Input: part model. Units: mm. Frame: model coordinates. Face numbers are marked on the shaded views. A direction names the side the tool comes from. Round coordinates to 2 decimals unless told otherwise and drop trailing zeros. Write each loop counter-clockwise with the first axis right and the second up, starting at its lowest first coordinate (ties: lowest second). Pieces come first, ordered by that corner, then holes. Notation, with made-up numbers: (64, 57) - (98, 57) arc R25 cw to (98, 88) - close; hole circle Ø9 at (30.25, 23.5). An arc over 180 degrees is marked (long way). Use one line per item in the form item = value.
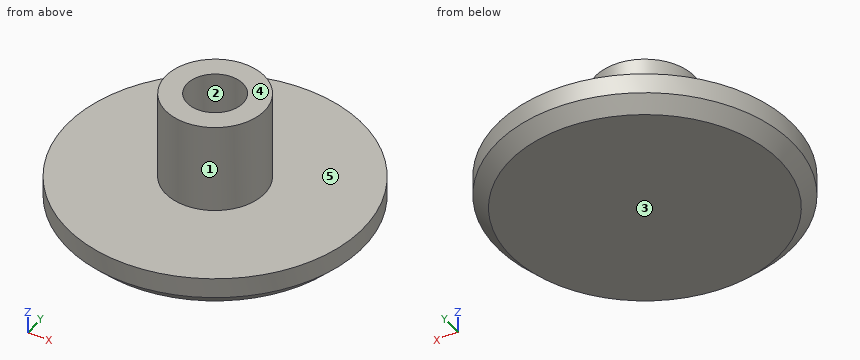
```python
from build123d import *

# Parameters (mm, degrees)
F0_R     = 11
F1_DEPTH = 2.5
F2_SIZE2 = 1
F2_SIZE  = 1
F3_R     = 3.675
F4_DEPTH = 6.6
F5_R     = 2.075
F6_DEPTH = 6


with BuildPart() as f1:
    # F0 (on Top) → F1 (new body)
    with BuildSketch(Plane.XY):
        Circle(F0_R)
    extrude(amount=F1_DEPTH)

    # F2
    f2_edges = [f1.edges().sort_by_distance(p)[0] for p in [
        (-11, 0, 0),
    ]]
    chamfer(f2_edges, length=F2_SIZE, length2=F2_SIZE2)

    # F3 (on face) → F4 (join)
    with BuildSketch(Plane.XY.offset(2.5)):
        Circle(F3_R)
    extrude(amount=F4_DEPTH)

    # F5 (on face) → F6 (cut)
    with BuildSketch(Plane.XY.offset(9.1)):
        Circle(F5_R)
    extrude(amount=-F6_DEPTH, mode=Mode.SUBTRACT)


solid = f1.part
```
(1) Draft query along Y for the marked faces 1, 2 and 3. Return one class per face: released by +Y, released by -Y, zero draft, split by the parting line, or undercut.
Derived:
face_1 = split by the parting line
face_2 = undercut
face_3 = zero draft
(2) Cut plane A-A on y = 0. Output: boundary loops of the cut face in (x, z) (3 decimals).
Derived:
outline = (-11, 1) - (-10, 0) - (10, 0) - (11, 1) - (11, 2.5) - (3.675, 2.5) - (3.675, 9.1) - (2.075, 9.1) - (2.075, 3.1) - (-2.075, 3.1) - (-2.075, 9.1) - (-3.675, 9.1) - (-3.675, 2.5) - (-11, 2.5) - close
(3) First-contact query: pin 1 Ø10 at (x, y) = (0, -7.5) entering from +Z; pin 2 Ø4 at (y, z) = (2, 5) entering from -X (3 decimals); pin 3 Ø1 at (y, z) = (2.5, 6) entering from -X; pin 4 Ø5 at (y, z) = (-6, 3) entering from -X. Flat tips, straight axial feed; report the tip coordinate or a pass-through.
Derived:
pin_1 = 9.1
pin_2 = -3.675
pin_3 = -3.08
pin_4 = -10.41
(4) Cut plane C-C on z = 4.5. Output: boundary loops of the cut face in (x, y) (3 decimals), then the cut area to 3 significant figures.
Derived:
outline = circle Ø7.35 at (0, 0); hole circle Ø4.15 at (0, 0)
area = 28.9 mm^2
(5) Material intervals for L1, parallel to Y at x = 0, z = 7.65 (3 decimals); L2, parallel to Z at x = -1.5, y = -4.5; L3, parallel to Y at x = 8.5, z = 2, sorted ascending.
Derived:
L1 = -3.675 to -2.075, 2.075 to 3.675
L2 = 0 to 2.5
L3 = -6.98 to 6.98
(6) Access query for the marked faces 4 and 5. Directions: +Z, -Z, +X, -X, +Y, -Y. A direction counts if a zero-diameter tool reaches every point of the face in a straight line with its end or side. Return the directions, or none.
Derived:
face_4 = +Z, +X, -X, +Y, -Y
face_5 = +Z
